```python
from build123d import *

# Parameters (mm, degrees)
ESQUISSE1_R                     = 28.2
BASE_EXTRUSION_DEPTH            = 45.97
BOSS_EXTRU_1_DEPTH              = 4.83
ESQUISSE3_R                     = 19.05
BOSS_EXTRU_2_DEPTH              = 1.52
ESQUISSE4_R                     = 2.54
ENL_V_MAT_EXTRU_1_DEPTH         = 65.584208596
ESQUISSE5_R                     = 3.175
ENL_V_MAT_EXTRU_2_DEPTH         = 30
R_P_TITION_LIN_AIRE1_COUNT      = 2
R_P_TITION_LIN_AIRE1_PITCH      = 47.1
R_P_TITION_LIN_AIRE1_COUNT_DIR2 = 2
R_P_TITION_LIN_AIRE1_PITCH_DIR2 = 47.1


with BuildPart() as part:
    # Esquisse1 → Base-Extrusion (new body)
    with BuildSketch(Plane.XY):
        Circle(ESQUISSE1_R)
    extrude(amount=BASE_EXTRUSION_DEPTH)

    # Esquisse2 → Boss.-Extru.1 (add)
    with BuildSketch(Plane.XY.offset(45.97)):
        with BuildLine():
            Line((-23.2, 28.2), (23.2, 28.2))
            ThreePointArc((23.2, 28.2), (26.735533906, 26.735533906), (28.2, 23.2))
            Line((28.2, 23.2), (28.2, -23.2))
            ThreePointArc((28.2, -23.2), (26.735533906, -26.735533906), (23.2, -28.2))
            Line((23.2, -28.2), (-23.2, -28.2))
            ThreePointArc((-23.2, -28.2), (-26.735533906, -26.735533906), (-28.2, -23.2))
            Line((-28.2, -23.2), (-28.2, 23.2))
            ThreePointArc((-28.2, 23.2), (-26.735533906, 26.735533906), (-23.2, 28.2))
        make_face()
    extrude(amount=BOSS_EXTRU_1_DEPTH)

    # Esquisse3 → Boss.-Extru.2 (add)
    with BuildSketch(Plane.XY.offset(50.8)):
        Circle(ESQUISSE3_R)
    extrude(amount=BOSS_EXTRU_2_DEPTH)

    # Esquisse4 → Enlèv. mat.-Extru.1 (cut, through all)
    with BuildSketch(Plane.XY.offset(50.8)):
        with Locations((-23.55, 23.55)):
            Circle(ESQUISSE4_R)
    enl_v_mat_extru_1 = extrude(amount=-ENL_V_MAT_EXTRU_1_DEPTH, mode=Mode.SUBTRACT)

    # Esquisse5 → Enlèv. mat.-Extru.2 (cut)
    with BuildSketch(Plane.XY.offset(52.32)):
        Circle(ESQUISSE5_R)
    extrude(amount=-ENL_V_MAT_EXTRU_2_DEPTH, mode=Mode.SUBTRACT)

    # Répétition linéaire1: Enl_v. mat.-Extru.1 2 × 2
    with Locations(*[(i * R_P_TITION_LIN_AIRE1_PITCH, -j * R_P_TITION_LIN_AIRE1_PITCH_DIR2, 0) for i in range(R_P_TITION_LIN_AIRE1_COUNT) for j in range(R_P_TITION_LIN_AIRE1_COUNT_DIR2) if (i, j) != (0, 0)]):
        add(enl_v_mat_extru_1, mode=Mode.SUBTRACT)


solid = part.part
```
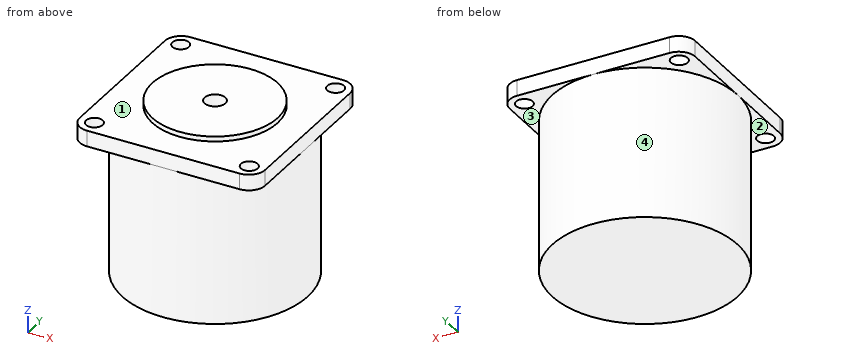
Model file for the job. Use its own axes, mm. Face numbers are marked on the shaded views. A direction names the side the tool comes from. Coordinates: 2 decimals unless noted, no trailing zeros. Loops run counter-clockwise (first coordinate to the right, second up) from the corner with the lowest first, then second, coordinate; pieces in that order, holes last. Notation, with made-up numbers: (-13, 40) - (12, 40) arc R25 cw to (12, 71) - close; hole circle Ø2 at (83.5, -3.75). An arc over 180 degrees is marked (long way). Answer as a JSON object with one key per item and string values. Group by question number.
(1) Cut at B-B (x = -6.5). Give the cut face in (y, z).
(2) Cut at C-C (z = 14). Give the cut face in (x, y), then the cut area to 3 significant figures.
(3) Cut at A-A (y = 22). Give the cut face in (x, z).
(4) Tool access for the marked faces 1, 2, 3 and 4: list every direction of +Z, -Z, +X, -X, +Y, -Y with a clear straight run to the whole face (end or side of a thin tool).
(5) Flat gauge pins, fed straight in: pin 1 (6 mm diameter, centred on x = -23.55, y = 23.55, fed in from -Z); pin 2 (8 mm diameter, centred on x = -19, z = 38.5, fed in from -Y); pin 3 (5 mm diameter, centred on y = -4, z = 32, fed in from -X). Where does each tip first touch, or does it go through?
(6) Probe line 1 along Y through (x, z) = (-23.55, 49.7); line 2 along X through (y, z) = (23, 49); line 3 along Z through (x, y) = (15.5, 17). List the from-to ranges inside material, lowest first.
(7) Cut at D-D (y = -5.5). Give the cut face in (x, z).
Geometry says:
{
 "1": {"outline": "(-28.2, 45.97) - (-27.44, 45.97) - (-27.44, 0) - (27.44, 0) - (27.44, 45.97) - (28.2, 45.97) - (28.2, 50.8) - (17.91, 50.8) - (17.91, 52.32) - (-17.91, 52.32) - (-17.91, 50.8) - (-28.2, 50.8) - close"},
 "2": {"outline": "circle Ø56.4 at (0, 0)", "area": "2,500 mm^2"},
 "3": {"outline": "(-28.2, 45.97) - (-25.56, 45.97) - (-25.56, 50.8) - (-28.2, 50.8) - close; (-21.54, 45.97) - (-17.64, 45.97) - (-17.64, 0) - (17.64, 0) - (17.64, 45.97) - (21.54, 45.97) - (21.54, 50.8) - (-21.54, 50.8) - close; (25.56, 45.97) - (28.2, 45.97) - (28.2, 50.8) - (25.56, 50.8) - close"},
 "4": {"face 1": "+Z", "face 2": "-Z, -X, -Y", "face 3": "-Z, +X, +Y", "face 4": "-Z"},
 "5": {"pin 1": "stops at z = 45.97", "pin 2": "stops at y = -23.88", "pin 3": "stops at x = -28.16"},
 "6": {"line 1": "y = -28.19 to -26.09, -21.01 to 21.01, 26.09 to 28.19", "line 2": "x = -28.2 to -26.03, -21.07 to 21.07, 26.03 to 28.2", "line 3": "z = 0 to 50.8"},
 "7": {"outline": "(-28.2, 45.97) - (-27.66, 45.97) - (-27.66, 0) - (27.66, 0) - (27.66, 45.97) - (28.2, 45.97) - (28.2, 50.8) - (18.24, 50.8) - (18.24, 52.32) - (-18.24, 52.32) - (-18.24, 50.8) - (-28.2, 50.8) - close"}
}
